Read the model definition and answer for the solid it produces. Units are mm, in the model's axes. Face numbers are marked on the shaded views. A direction names the side the tool comes from. Give positions to 0.01 mm unless a question says otherwise; leave off trailing zeros. Loops run counter-clockwise (first coordinate to the right, second up) from the corner with the lowest first, then second, coordinate; pieces in that order, holes last. Notation, with made-up numbers: (21.5, 67.25) - (53.5, 67.25) arc R28 cw to (53.5, 101.25) - close; hole circle Ø1 at (-35, -23.75). An arc over 180 degrees is marked (long way). Put each result on its own line as item: value. Start each with the question number.
1. Consider L1, parallel to Z at x = 0, y = -0.4; L2, parallel to X at y = -2.5, z = 1; L3, parallel to Z at x = 2.5, y = -1.75. Determine where each line is inside the solid, lowest interval first. Write a range as from..to.
2. A cutting plane is placed at B-B, the plane z = 0. Determine the outline of the cut face in (x, y) (3 decimals).
3. A cutting plane is placed at D-D, the plane x = -31.75. Determine the outline of the cut face in (y, z).
4. For the marked faces 1 and 2, determine the directions among +Z, -Z, +X, -X, +Y, -Y from which every point of the face is accessible in a straight line to the end or side of a thin tool.
5. Given pin 1 Ø5 at (x, z) = (-31.75, 0) entering from +Y; pin 2 Ø3 at (y, z) = (3.5, -29) entering from -X; pin 3 Ø2 at (y, z) = (-2.5, 4) entering from -X; pin 4 Ø1.5 at (x, z) = (28.5, -13.5) entering from +Y, each flat-ended and moving along its own axis, determine where each tip first touches the part or whether it passes through.
6. A cutting plane is placed at C-C, the plane y = 1.75. Determine the outline of the cut face in (x, z), plus the area to 3 significant figures.
7. A cutting plane is placed at A-A, the plane x = 0. Determine the outline of the cut face in (y, z) (3 decimals).
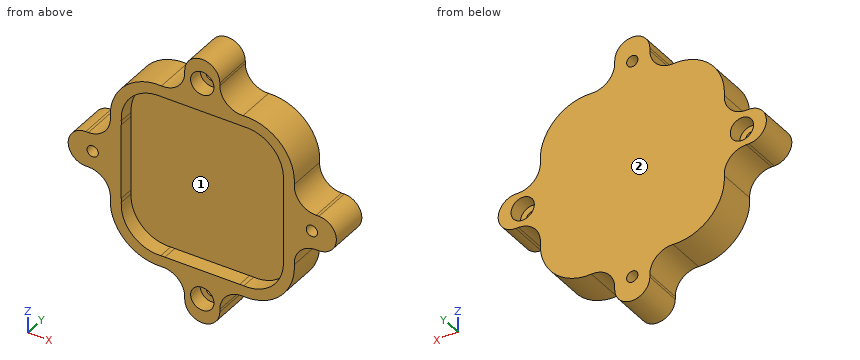
```python
from build123d import *

# Parameters (mm, degrees)
BOSS_EXTRUDE4_DEPTH                                 = 3.81
BOSS_EXTRUDE4_DEPTH_BACK                            = 7.62
CUT_EXTRUDE1_DEPTH                                  = 4.445
CBORE_FOR_4_BINDING_HEAD_MACHINE_SCREW3_D           = 3.2639
CBORE_FOR_4_BINDING_HEAD_MACHINE_SCREW3_CBORE_D     = 6.74624
CBORE_FOR_4_BINDING_HEAD_MACHINE_SCREW3_CBORE_DEPTH = 4.2672
CBORE_FOR_4_BINDING_HEAD_MACHINE_SCREW4_D           = 3.2639
CBORE_FOR_4_BINDING_HEAD_MACHINE_SCREW4_CBORE_D     = 6.74624
CBORE_FOR_4_BINDING_HEAD_MACHINE_SCREW4_CBORE_DEPTH = 4.2672


with BuildPart() as part:
    # Sketch5 → Boss-Extrude4 (new, two sides: drawn at the far end of the back side and taken through both)
    with BuildSketch(Plane(origin=(0, 0, 0), x_dir=(-1, 0, 0), z_dir=(0, -1, 0)).offset(-BOSS_EXTRUDE4_DEPTH_BACK)):
        with BuildLine():
            Line((33.759871133, -5.08), (32.980273667, -5.08))
            ThreePointArc((32.980273667, -5.08), (28.3519556, -7.0824522), (26.642688146, -11.826875))
            ThreePointArc((26.642688146, -11.826875), (22.578281733, -22.578281733), (11.826875, -26.642688146))
            ThreePointArc((11.826875, -26.642688146), (7.0824522, -28.3519556), (5.08, -32.980273667))
            Line((5.08, -32.980273667), (5.08, -33.759871133))
            ThreePointArc((5.08, -33.759871133), (0, -38.839871133), (-5.08, -33.759871133))
            Line((-5.08, -33.759871133), (-5.08, -32.980273667))
            ThreePointArc((-5.08, -32.980273667), (-7.0824522, -28.3519556), (-11.826875, -26.642688146))
            ThreePointArc((-11.826875, -26.642688146), (-22.578281733, -22.578281733), (-26.642688146, -11.826875))
            ThreePointArc((-26.642688146, -11.826875), (-28.3519556, -7.0824522), (-32.980273667, -5.08))
            Line((-32.980273667, -5.08), (-33.759871133, -5.08))
            ThreePointArc((-33.759871133, -5.08), (-38.839871133, 0), (-33.759871133, 5.08))
            Line((-33.759871133, 5.08), (-32.980273667, 5.08))
            ThreePointArc((-32.980273667, 5.08), (-28.3519556, 7.0824522), (-26.642688146, 11.826875))
            ThreePointArc((-26.642688146, 11.826875), (-22.578281733, 22.578281733), (-11.826875, 26.642688146))
            ThreePointArc((-11.826875, 26.642688146), (-7.0824522, 28.3519556), (-5.08, 32.980273667))
            Line((-5.08, 32.980273667), (-5.08, 33.759871133))
            ThreePointArc((-5.08, 33.759871133), (0, 38.839871133), (5.08, 33.759871133))
            Line((5.08, 33.759871133), (5.08, 32.980273667))
            ThreePointArc((5.08, 32.980273667), (7.0824522, 28.3519556), (11.826875, 26.642688146))
            ThreePointArc((11.826875, 26.642688146), (22.578281733, 22.578281733), (26.642688146, 11.826875))
            ThreePointArc((26.642688146, 11.826875), (28.3519556, 7.0824522), (32.980273667, 5.08))
            Line((32.980273667, 5.08), (33.759871133, 5.08))
            ThreePointArc((33.759871133, 5.08), (38.839871133, 0), (33.759871133, -5.08))
        make_face()
    extrude(amount=BOSS_EXTRUDE4_DEPTH + BOSS_EXTRUDE4_DEPTH_BACK)

    # Sketch21 → Cut-Extrude1 (cut)
    with BuildSketch(Plane.XZ.offset(3.81)):
        with BuildLine():
            ThreePointArc((23.473895385, 12.0253125), (20.333217703, 20.333217703), (12.0253125, 23.473895385))
            ThreePointArc((12.0253125, 23.473895385), (11.43, 23.455273667), (10.8346875, 23.473895385))
            Line((10.8346875, 23.473895385), (-10.8346875, 23.473895385))
            ThreePointArc((-10.8346875, 23.473895385), (-11.43, 23.455273667), (-12.0253125, 23.473895385))
            ThreePointArc((-12.0253125, 23.473895385), (-20.333217703, 20.333217703), (-23.473895385, 12.0253125))
            ThreePointArc((-23.473895385, 12.0253125), (-23.455273667, 11.43), (-23.473895385, 10.8346875))
            Line((-23.473895385, 10.8346875), (-23.473895385, -10.8346875))
            ThreePointArc((-23.473895385, -10.8346875), (-23.455273667, -11.43), (-23.473895385, -12.0253125))
            ThreePointArc((-23.473895385, -12.0253125), (-20.333217703, -20.333217703), (-12.0253125, -23.473895385))
            ThreePointArc((-12.0253125, -23.473895385), (-11.43, -23.455273667), (-10.8346875, -23.473895385))
            Line((-10.8346875, -23.473895385), (10.8346875, -23.473895385))
            ThreePointArc((10.8346875, -23.473895385), (11.43, -23.455273667), (12.0253125, -23.473895385))
            ThreePointArc((12.0253125, -23.473895385), (20.333217703, -20.333217703), (23.473895385, -12.0253125))
            ThreePointArc((23.473895385, -12.0253125), (23.455273667, -11.43), (23.473895385, -10.8346875))
            Line((23.473895385, -10.8346875), (23.473895385, 10.8346875))
            ThreePointArc((23.473895385, 10.8346875), (23.455273667, 11.43), (23.473895385, 12.0253125))
        make_face()
    extrude(amount=-CUT_EXTRUDE1_DEPTH, mode=Mode.SUBTRACT)

    # CBORE for #4 Binding Head Machine Screw3 (through all)
    with Locations(Plane(origin=(0, -3.81, 0), x_dir=(-1, 0, 0), z_dir=(0, -1, 0))):
        with Locations((0, 31.75), (0, -31.75)):
            CounterBoreHole(CBORE_FOR_4_BINDING_HEAD_MACHINE_SCREW3_D / 2, CBORE_FOR_4_BINDING_HEAD_MACHINE_SCREW3_CBORE_D / 2, CBORE_FOR_4_BINDING_HEAD_MACHINE_SCREW3_CBORE_DEPTH)

    # CBORE for #4 Binding Head Machine Screw4 (through all)
    with Locations(Plane(origin=(0, 7.62, 0), x_dir=(1, 0, 0), z_dir=(0, 1, 0))):
        with Locations((31.75, 0), (-31.75, 0)):
            CounterBoreHole(CBORE_FOR_4_BINDING_HEAD_MACHINE_SCREW4_D / 2, CBORE_FOR_4_BINDING_HEAD_MACHINE_SCREW4_CBORE_D / 2, CBORE_FOR_4_BINDING_HEAD_MACHINE_SCREW4_CBORE_DEPTH)


solid = part.part
```
Return value:
1. L1: z = -38.84..-35.12, -28.38..-23.47, 23.47..28.38, 35.12..38.84
1. L2: x = -38.74..-33.04, -30.46..-23.47, 23.47..30.46, 33.04..38.74
1. L3: z = -38.18..-34.01, -29.49..-23.47, 23.47..29.49, 34.01..38.18
2. outline: (-38.84, -3.81) - (-33.382, -3.81) - (-33.382, 3.353) - (-35.123, 3.353) - (-35.123, 7.62) - (-38.84, 7.62) - close; (-30.118, -3.81) - (-23.474, -3.81) - (-23.474, 0.635) - (23.474, 0.635) - (23.474, -3.81) - (30.118, -3.81) - (30.118, 3.353) - (28.377, 3.353) - (28.377, 7.62) - (-28.377, 7.62) - (-28.377, 3.353) - (-30.118, 3.353) - close; (33.382, -3.81) - (38.84, -3.81) - (38.84, 7.62) - (35.123, 7.62) - (35.123, 3.353) - (33.382, 3.353) - close
3. outline: (-3.81, -5.2) - (7.62, -5.2) - (7.62, -3.37) - (3.35, -3.37) - (3.35, -1.63) - (-3.81, -1.63) - close; (-3.81, 1.63) - (3.35, 1.63) - (3.35, 3.37) - (7.62, 3.37) - (7.62, 5.2) - (-3.81, 5.2) - close
4. face 1: -Y
4. face 2: +Z, -Z, +X, -X, +Y
5. pin 1: stops at y = 3.35
5. pin 2: stops at x = -8.22
5. pin 3: stops at x = -37.86
5. pin 4: passes through
6. outline: (-33.76, -5.08) - (-32.98, -5.08) arc R6.35 cw to (-26.64, -11.83) arc R13.97 ccw to (-11.83, -26.64) arc R6.35 cw to (-5.08, -32.98) - (-5.08, -33.76) arc R5.08 ccw to (5.08, -33.76) - (5.08, -32.98) arc R6.35 cw to (11.83, -26.64) arc R13.97 ccw to (26.64, -11.83) arc R6.35 cw to (32.98, -5.08) - (33.76, -5.08) arc R5.08 ccw to (33.76, 5.08) - (32.98, 5.08) arc R6.35 cw to (26.64, 11.83) arc R13.97 ccw to (11.83, 26.64) arc R6.35 cw to (5.08, 32.98) - (5.08, 33.76) arc R5.08 ccw to (-5.08, 33.76) - (-5.08, 32.98) arc R6.35 cw to (-11.83, 26.64) arc R13.97 ccw to (-26.64, 11.83) arc R6.35 cw to (-32.98, 5.08) - (-33.76, 5.08) arc R5.08 ccw to start; hole circle Ø3.26 at (-31.75, 0); hole circle Ø3.26 at (0, -31.75); hole circle Ø3.26 at (0, 31.75); hole circle Ø3.26 at (31.75, 0)
6. area: 3,160 mm2
7. outline: (-3.81, -38.84) - (7.62, -38.84) - (7.62, -33.382) - (0.457, -33.382) - (0.457, -35.123) - (-3.81, -35.123) - close; (-3.81, -28.377) - (0.457, -28.377) - (0.457, -30.118) - (7.62, -30.118) - (7.62, 30.118) - (0.457, 30.118) - (0.457, 28.377) - (-3.81, 28.377) - (-3.81, 23.474) - (0.635, 23.474) - (0.635, -23.474) - (-3.81, -23.474) - close; (-3.81, 35.123) - (0.457, 35.123) - (0.457, 33.382) - (7.62, 33.382) - (7.62, 38.84) - (-3.81, 38.84) - close
